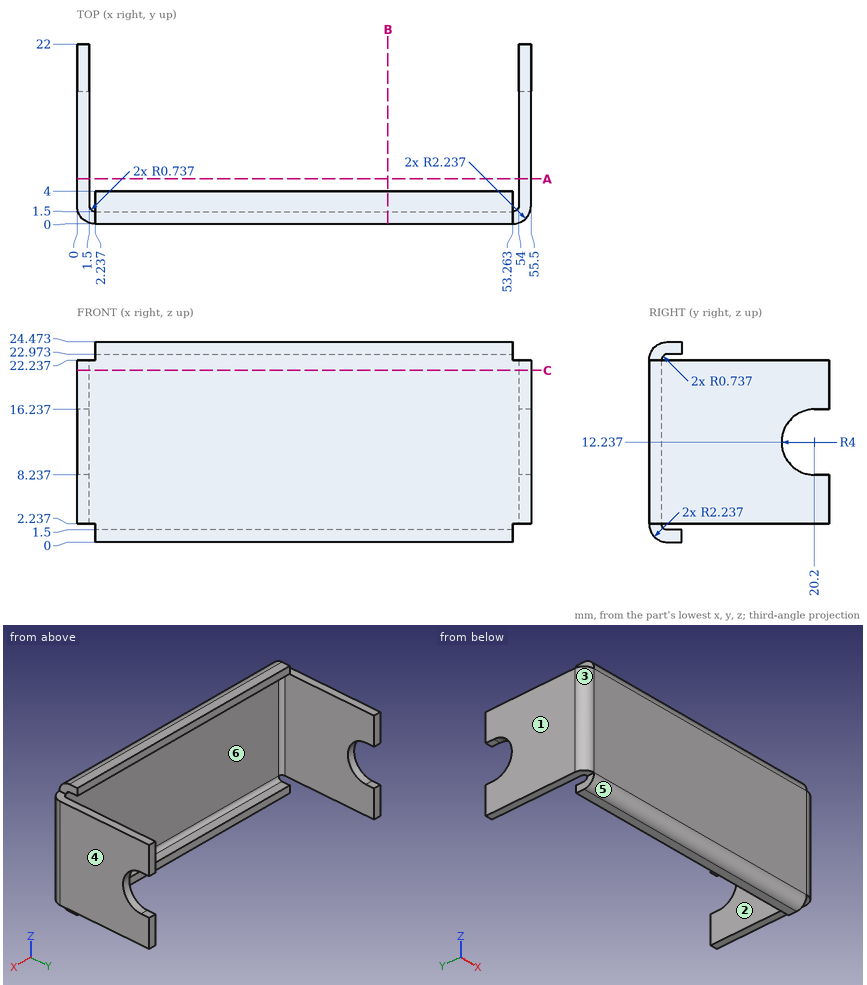
Input: dimensioned drawing with shaded views. Units: mm. Origin: part minimum x, y, z. A direction names the side the tool comes from. Give positions to 0.01 mm unless a question says otherwise; leave off trailing zeros. Write each loop counter-clockwise with the first axis right and the second up, starting at its lowest first coordinate (ties: lowest second). Pieces come first, ordered by that corner, then holes. Notation, with made-up numbers: (81, -19) -> (134, -19) arc R12 cw to (134, 0) -> close; hole circle Ø11 at (-26.75, 35.25). An arc over 180 degrees is marked (long way). Answer as a JSON object with one key per item and string values.
1. Ray query, probe 1 along X at (y, z) = (18.5, 6.5); probe 2 along Y at (x, z) = (13.5, 9); probe 3 along X at (y, z) = (1.75, 5.25) (1 decimal). Return the intervals inside material, ascending. Write a range as from..to.
Ans:
{"probe 1": "x = 0..1.5, 54..55.5", "probe 2": "y = 0..1.5", "probe 3": "x = 0.1..1.7, 53.8..55.4"}
2. Mould query, pull axis X, two halves, no side actions, for the marked faces 3, 4, 5 and 6. Classes: pulls with the +X half, pulls with the -X half, needs draft (parallel to the pull), parting line crosses it, or undercut.
Ans:
{"face 3": "pulls with the -X half", "face 4": "pulls with the +X half", "face 5": "needs draft", "face 6": "undercut"}
3. Cut plane A-A on y = 5.5. Output: boundary loops of the cut face in (x, z).
Ans:
{"outline": "(0, 2.24) -> (1.5, 2.24) -> (1.5, 22.24) -> (0, 22.24) -> close; (54, 2.24) -> (55.5, 2.24) -> (55.5, 22.24) -> (54, 22.24) -> close"}
4. Cut plane B-B on x = 38. Output: boundary loops of the cut face in (y, z).
Ans:
{"outline": "(0, 2.24) arc R2.24 ccw to (2.24, 0) -> (4, 0) -> (4, 1.5) -> (2.24, 1.5) arc R0.74 cw to (1.5, 2.24) -> (1.5, 22.24) arc R0.74 cw to (2.24, 22.97) -> (4, 22.97) -> (4, 24.47) -> (2.24, 24.47) arc R2.24 ccw to (0, 22.24) -> close"}
5. Contact query for flat-ended pins moving along their axis: pin 1 (12 mm diameter, centred on x = 42.5, z = 19.5, fed in from +Y); pin 2 (1.8 mm diameter, centred on x = 1.5, y = 16.5, fed in from -Z); pin 3 (0.7 mm diameter, centred on y = 3, z = 23.5, fed in from +X); pin 4 (10 mm diameter, centred on x = 23, y = 9.5, fed in from +Z). Output: stop coordinate, or through.
Ans:
{"pin 1": "stops at y = 4", "pin 2": "stops at z = 2.24", "pin 3": "stops at x = 53.26", "pin 4": "passes through"}
6. Cut plane C-C on z = 21. Output: boundary loops of the cut face in (x, y).
Ans:
{"outline": "(0, 2.24) arc R2.24 ccw to (2.24, 0) -> (53.26, 0) arc R2.24 ccw to (55.5, 2.24) -> (55.5, 22) -> (54, 22) -> (54, 2.24) arc R0.74 cw to (53.26, 1.5) -> (2.24, 1.5) arc R0.74 cw to (1.5, 2.24) -> (1.5, 22) -> (0, 22) -> close"}
7. Access query for the marked faces 1 and 2. Directions: +Z, -Z, +X, -X, +Y, -Y. A direction counts if a zero-diameter tool reaches every point of the face in a straight line with its end or side. Return the directions, or none.
Ans:
{"face 1": "+Z, -Z, -X, +Y, -Y", "face 2": "+Z, -Z, +Y"}
